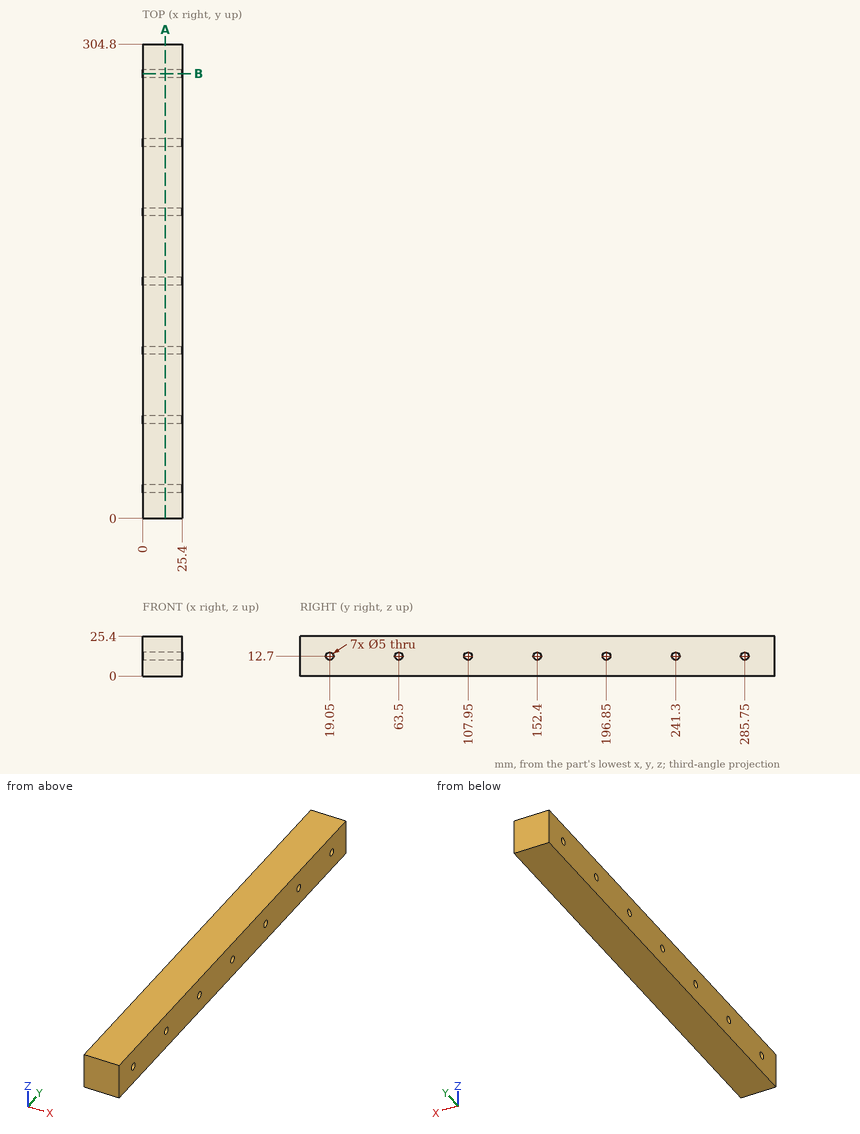
Geometry: see drawing. Coordinates: mm, zero at the bounding-box minimum. Coordinates: 2 decimals unless noted, no trailing zeros. Order: outer loops, then holes, each group sorted by start corner. A loop starts at its lowest first (then second) coordinate and runs counter-clockwise, first axis right, second up. Notation, with made-up numbers: M -32.5,-31.5 L -10.5,-31.5 A25 cw -10.5,-3.5 Z; hole C 87,23 d11. An arc over 180 degrees is marked long. Write item = value, one per line. Start each with the question number.
(1) Line query: line 1 along Z through (x, y) = (14.5, 152.4); line 2 along Z through (x, y) = (2.25, 239.5). Output: solid intervals per line, ascending. Write a range as [from, to].
(2) Section A-A on x = 14.75. Output: boundary loops of the cut face in (y, z), and give its area (3 significant figures).
(3) First-contact query: P1, Ø6.5, axis at y = 241.3, z = 12.7, coming from the -X side. Flat tip, straight axial feed; report the tip coordinate or a pass-through.
(4) Section B-B on y = 285.75. Output: boundary loops of the cut face in (x, z).
Result set:
q1.line_1 = [0, 10.2], [15.2, 25.4]
q1.line_2 = [0, 10.97], [14.43, 25.4]
q2.outline = M 0,0 L 304.8,0 L 304.8,25.4 L 0,25.4 Z; hole C 19.05,12.7 d5; hole C 63.5,12.7 d5; hole C 107.95,12.7 d5; hole C 152.4,12.7 d5; hole C 196.85,12.7 d5; hole C 241.3,12.7 d5; hole C 285.75,12.7 d5
q2.area = 7,600 mm²
q3.P1 = 0
q4.outline = M 0,0 L 25.4,0 L 25.4,10.2 L 0,10.2 Z; M 0,15.2 L 25.4,15.2 L 25.4,25.4 L 0,25.4 Z
